```python
from build123d import *

# Parameters (mm, degrees)
F1_DEPTH = 6.3
F2_SIZE  = 0.5
F3_SIZE  = 2
F4_W     = 10
F4_H     = 0.938
F4_H_2   = 5.5
F5_DEPTH = 2.5
F6_SIZE  = 1
F7_SIZE  = 2


# Not quite as in the source:
# - a feature names something its author has since deleted; it is built from what else it names


with BuildPart() as f1:
    # F0 (on Top) → F1 (new body)
    with BuildSketch(Plane.XY):
        with BuildLine():
            ThreePointArc((27, -22.5), (49.5, 0), (27, 22.5))
            Line((27, 22.5), (27, 4))
            Line((27, 4), (34.5, 4))
            ThreePointArc((34.5, 4), (38.5, 0), (34.5, -4))
            Line((34.5, -4), (27, -4))
            Line((27, -4), (27, -22.5))
        make_face()
        with BuildLine():
            ThreePointArc((30.8505792452, -11.1005792452), (28.6005792452, -8.8505792452), (30.8505792452, -6.6005792452))
            Line((30.8505792452, -6.6005792452), (40.8505792452, -6.6005792452))
            ThreePointArc((40.8505792452, -6.6005792452), (43.1005792452, -8.8505792452), (40.8505792452, -11.1005792452))
            Line((40.8505792452, -11.1005792452), (30.8505792452, -11.1005792452))
        make_face(mode=Mode.SUBTRACT)
        with BuildLine():
            ThreePointArc((30.8505792452, 6.6005792452), (28.6005792452, 8.8505792452), (30.8505792452, 11.1005792452))
            Line((30.8505792452, 11.1005792452), (40.8505792452, 11.1005792452))
            ThreePointArc((40.8505792452, 11.1005792452), (43.1005792452, 8.8505792452), (40.8505792452, 6.6005792452))
            Line((40.8505792452, 6.6005792452), (30.8505792452, 6.6005792452))
        make_face(mode=Mode.SUBTRACT)
        with BuildLine():
            Line((27, 4), (27, 22.5))
            Line((27, 22.5), (-27, 22.5))
            Line((-27, 22.5), (-27, 8.905))
            ThreePointArc((-27, 8.905), (-20.7032141135, 6.2967858865), (-18.095, 0))
            ThreePointArc((-18.095, 0), (-20.7032141135, -6.2967858865), (-27, -8.905))
            Line((-27, -8.905), (-27, -22.5))
            Line((-27, -22.5), (27, -22.5))
            Line((27, -22.5), (27, -4))
            Line((27, -4), (19.5, -4))
            ThreePointArc((19.5, -4), (15.5, 0), (19.5, 4))
            Line((19.5, 4), (27, 4))
        make_face()
        with BuildLine():
            Line((23.1494207548, -11.1005792452), (13.1494207548, -11.1005792452))
            ThreePointArc((13.1494207548, -11.1005792452), (10.8994207548, -8.8505792452), (13.1494207548, -6.6005792452))
            Line((13.1494207548, -6.6005792452), (23.1494207548, -6.6005792452))
            ThreePointArc((23.1494207548, -6.6005792452), (25.3994207548, -8.8505792452), (23.1494207548, -11.1005792452))
        make_face(mode=Mode.SUBTRACT)
        with BuildLine():
            ThreePointArc((13.1494207548, 6.6005792452), (10.8994207548, 8.8505792452), (13.1494207548, 11.1005792452))
            Line((13.1494207548, 11.1005792452), (23.1494207548, 11.1005792452))
            ThreePointArc((23.1494207548, 11.1005792452), (25.3994207548, 8.8505792452), (23.1494207548, 6.6005792452))
            Line((23.1494207548, 6.6005792452), (13.1494207548, 6.6005792452))
        make_face(mode=Mode.SUBTRACT)
        with BuildLine():
            Line((-27, 8.905), (-27, 22.5))
            ThreePointArc((-27, 22.5), (-49.5, 0), (-27, -22.5))
            Line((-27, -22.5), (-27, -8.905))
            ThreePointArc((-27, -8.905), (-35.905, 0), (-27, 8.905))
        make_face()
    extrude(amount=F1_DEPTH)

    # F2
    f2_edges = [f1.edges().sort_by_distance(p)[0] for p in [
        (18.149421, 11.100579, 6.3),
        (35.850579, 11.100579, 6.3),
        (35.850579, -6.600579, 6.3),
        (18.149421, -6.600579, 6.3),
        (35.850579, 11.100579, 0),
        (18.149421, 11.100579, 0),
        (35.850579, -6.600579, 0),
        (18.149421, -6.600579, 0),
        (43.100579, -8.850579, 0),
        (35.850579, -11.100579, 0),
        (28.600579, -8.850579, 0),
        (43.100579, 8.850579, 0),
        (35.850579, 6.600579, 0),
        (28.600579, 8.850579, 0),
        (18.149421, 6.600579, 0),
        (10.899421, 8.850579, 0),
        (25.399421, 8.850579, 0),
        (18.149421, -11.100579, 0),
        (10.899421, -8.850579, 0),
        (25.399421, -8.850579, 0),
    ]]
    chamfer(f2_edges, length=F2_SIZE)

    # F3
    f3_edges = [f1.edges().sort_by_distance(p)[0] for p in [
        (0, -22.5, 6.3),
        (0, -22.5, 0),
    ]]
    chamfer(f3_edges, length=F3_SIZE)

    # F4 (on face) → F5 (cut)
    with BuildSketch(Plane.XY.offset(6.3)):
        with Locations((18.1494207548, 12.0695792452)):
            Rectangle(F4_W, F4_H)
        with BuildLine():
            Line((13.1494207548, 11.6005792452), (13.1494207548, 12.5385792452))
            ThreePointArc((13.1494207548, 12.5385792452), (9.4614207548, 8.8505792452), (13.1494207548, 5.1625792452))
            Line((13.1494207548, 5.1625792452), (13.1494207548, 6.1005792452))
            ThreePointArc((13.1494207548, 6.1005792452), (10.3994207548, 8.8505792452), (13.1494207548, 11.6005792452))
        make_face()
        with BuildLine():
            Line((13.1494207548, 6.1005792452), (13.1494207548, 11.6005792452))
            ThreePointArc((13.1494207548, 11.6005792452), (10.3994207548, 8.8505792452), (13.1494207548, 6.1005792452))
        make_face()
        with Locations((18.1494207548, 8.8505792452)):
            Rectangle(F4_W, F4_H_2)
        with Locations((18.1494207548, 5.6315792452)):
            Rectangle(F4_W, F4_H)
        with BuildLine():
            ThreePointArc((23.1494207548, 6.1005792452), (25.8994207548, 8.8505792452), (23.1494207548, 11.6005792452))
            Line((23.1494207548, 11.6005792452), (23.1494207548, 6.1005792452))
        make_face()
        with BuildLine():
            ThreePointArc((23.1494207548, 5.1625792452), (26.8374207548, 8.8505792452), (23.1494207548, 12.5385792452))
            Line((23.1494207548, 12.5385792452), (23.1494207548, 11.6005792452))
            ThreePointArc((23.1494207548, 11.6005792452), (25.8994207548, 8.8505792452), (23.1494207548, 6.1005792452))
            Line((23.1494207548, 6.1005792452), (23.1494207548, 5.1625792452))
        make_face()
        with BuildLine():
            ThreePointArc((30.8505792452, 12.5385792452), (27.1625792452, 8.8505792452), (30.8505792452, 5.1625792452))
            Line((30.8505792452, 5.1625792452), (30.8505792452, 6.1005792452))
            ThreePointArc((30.8505792452, 6.1005792452), (28.1005792452, 8.8505792452), (30.8505792452, 11.6005792452))
            Line((30.8505792452, 11.6005792452), (30.8505792452, 12.5385792452))
        make_face()
        with BuildLine():
            ThreePointArc((30.8505792452, 11.6005792452), (28.1005792452, 8.8505792452), (30.8505792452, 6.1005792452))
            Line((30.8505792452, 6.1005792452), (30.8505792452, 11.6005792452))
        make_face()
        with Locations((35.8505792452, 8.8505792452)):
            Rectangle(F4_W, F4_H_2)
        with Locations((35.8505792452, 12.0695792452)):
            Rectangle(F4_W, F4_H)
        with Locations((35.8505792452, 5.6315792452)):
            Rectangle(F4_W, F4_H)
        with BuildLine():
            Line((40.8505792452, 6.1005792452), (40.8505792452, 5.1625792452))
            ThreePointArc((40.8505792452, 5.1625792452), (44.5385792452, 8.8505792452), (40.8505792452, 12.5385792452))
            Line((40.8505792452, 12.5385792452), (40.8505792452, 11.6005792452))
            ThreePointArc((40.8505792452, 11.6005792452), (43.6005792452, 8.8505792452), (40.8505792452, 6.1005792452))
        make_face()
        with BuildLine():
            Line((40.8505792452, 11.6005792452), (40.8505792452, 6.1005792452))
            ThreePointArc((40.8505792452, 6.1005792452), (43.6005792452, 8.8505792452), (40.8505792452, 11.6005792452))
        make_face()
        with Locations((18.1494207548, -8.8505792452)):
            Rectangle(F4_W, F4_H_2)
        with BuildLine():
            ThreePointArc((13.1494207548, -6.1005792452), (10.3994207548, -8.8505792452), (13.1494207548, -11.6005792452))
            Line((13.1494207548, -11.6005792452), (13.1494207548, -6.1005792452))
        make_face()
        with BuildLine():
            Line((23.1494207548, -6.1005792452), (23.1494207548, -11.6005792452))
            ThreePointArc((23.1494207548, -11.6005792452), (25.8994207548, -8.8505792452), (23.1494207548, -6.1005792452))
        make_face()
        with Locations((18.1494207548, -5.6315792452)):
            Rectangle(F4_W, F4_H)
        with BuildLine():
            Line((23.1494207548, -11.6005792452), (23.1494207548, -12.5385792452))
            ThreePointArc((23.1494207548, -12.5385792452), (26.8374207548, -8.8505792452), (23.1494207548, -5.1625792452))
            Line((23.1494207548, -5.1625792452), (23.1494207548, -6.1005792452))
            ThreePointArc((23.1494207548, -6.1005792452), (25.8994207548, -8.8505792452), (23.1494207548, -11.6005792452))
        make_face()
        with Locations((18.1494207548, -12.0695792452)):
            Rectangle(F4_W, F4_H)
        with BuildLine():
            ThreePointArc((13.1494207548, -5.1625792452), (9.4614207548, -8.8505792452), (13.1494207548, -12.5385792452))
            Line((13.1494207548, -12.5385792452), (13.1494207548, -11.6005792452))
            ThreePointArc((13.1494207548, -11.6005792452), (10.3994207548, -8.8505792452), (13.1494207548, -6.1005792452))
            Line((13.1494207548, -6.1005792452), (13.1494207548, -5.1625792452))
        make_face()
        with BuildLine():
            ThreePointArc((30.8505792452, -5.1625792452), (27.1625792452, -8.8505792452), (30.8505792452, -12.5385792452))
            Line((30.8505792452, -12.5385792452), (30.8505792452, -11.6005792452))
            ThreePointArc((30.8505792452, -11.6005792452), (28.1005792452, -8.8505792452), (30.8505792452, -6.1005792452))
            Line((30.8505792452, -6.1005792452), (30.8505792452, -5.1625792452))
        make_face()
        with Locations((35.8505792452, -5.6315792452)):
            Rectangle(F4_W, F4_H)
        with Locations((35.8505792452, -8.8505792452)):
            Rectangle(F4_W, F4_H_2)
        with Locations((35.8505792452, -12.0695792452)):
            Rectangle(F4_W, F4_H)
        with BuildLine():
            ThreePointArc((30.8505792452, -6.1005792452), (28.1005792452, -8.8505792452), (30.8505792452, -11.6005792452))
            Line((30.8505792452, -11.6005792452), (30.8505792452, -6.1005792452))
        make_face()
        with BuildLine():
            Line((40.8505792452, -6.1005792452), (40.8505792452, -11.6005792452))
            ThreePointArc((40.8505792452, -11.6005792452), (43.6005792452, -8.8505792452), (40.8505792452, -6.1005792452))
        make_face()
        with BuildLine():
            Line((40.8505792452, -11.6005792452), (40.8505792452, -12.5385792452))
            ThreePointArc((40.8505792452, -12.5385792452), (44.5385792452, -8.8505792452), (40.8505792452, -5.1625792452))
            Line((40.8505792452, -5.1625792452), (40.8505792452, -6.1005792452))
            ThreePointArc((40.8505792452, -6.1005792452), (43.6005792452, -8.8505792452), (40.8505792452, -11.6005792452))
        make_face()
    extrude(amount=-F5_DEPTH, mode=Mode.SUBTRACT)

    # F6
    f6_edges = [f1.edges().sort_by_distance(p)[0] for p in [
        (10.899421, 8.850579, 3.8),
        (18.149421, 6.600579, 3.8),
        (25.399421, 8.850579, 3.8),
        (18.149421, 11.100579, 3.8),
        (35.850579, 11.100579, 3.8),
        (28.600579, 8.850579, 3.8),
        (43.100579, 8.850579, 3.8),
        (35.850579, 6.600579, 3.8),
        (35.850579, -6.600579, 3.8),
        (28.600579, -8.850579, 3.8),
        (43.100579, -8.850579, 3.8),
        (35.850579, -11.100579, 3.8),
        (18.149421, -6.600579, 3.8),
        (10.899421, -8.850579, 3.8),
        (25.399421, -8.850579, 3.8),
        (18.149421, -11.100579, 3.8),
    ]]
    chamfer(f6_edges, length=F6_SIZE)

    # F7
    f7_edges = [f1.edges().sort_by_distance(p)[0] for p in [
        (27, 4, 0),
        (38.5, 0, 0),
        (27, -4, 0),
        (15.5, 0, 0),
    ]]
    chamfer(f7_edges, length=F7_SIZE)


solid = f1.part
```
Model file for the job. Use its own axes, mm. A direction names the side the tool comes from. Give positions to 0.01 mm unless a question says otherwise; leave off trailing zeros. Order: outer loops, then holes, each group sorted by start corner. A loop starts at its lowest first (then second) coordinate and runs counter-clockwise, first axis right, second up.
1) Saw through at A-A, the plane z = 5.25. Write the cut outline in (x, y) (3 decimals).
2) Wall check: probe 1 along X at (y, z) = (-10.5, 4.5); probe 2 along Y at (x, z) = (33, 6.25); probe 3 along X at (y, z) = (-11, 6.25). Give the ranges that are in metal, low to high.
3) Pin check, flat tips, straight feed: pin 1 (0.8 mm diameter, centred on x = 20, z = 5, fed in from +Y); pin 2 (6 mm diameter, centred on x = 17, y = 9, fed in from +Z); pin 3 (3.5 mm diameter, centred on x = 36, y = -10, fed in from +Z). Stop position of each tip, or through.
4) Mould opens along X. For faces 5 (the flat face through (18, 11.101, 2)), 6 (the cylindrical face through (38.5, 0.1, 4.1)), 7 (the flat face through (-1, 0, 6.3)), 8 (the conical face through (47.62, -0.454, 0.125)) say: +X half, -X half, draft (parallel to the pull), parting line (faces both ways), or undercut.
5) Saw through at B-B, the plane x = -25. Write the cut outline in (y, z).
6) 3-axis set-ups, long thin cutter, end or side, ignore diameter. For faces 1 (the flat face through (18, -5.163, 5)), 2 (the flat face through (0, -22.5, 3)), 3 (the conical face through (38.8, 0.1, 1.7)), 4 (the cylindrical face through (43.1, 8.9, 1.6)): which of +Z, -Z, +X, -X, +Y, -Y reach the whole face in a straight line?
7) Saw through at C-C, the plane x = 35.5. Count the separate pieces of the cut face and the enclosed holes in it, then the cut area to 3 significant figures.
Computed:
1. outline: (-27, -21.55) - (27, -21.55) arc R21.55 ccw to (27, 21.55) - (-27, 21.55) arc R21.55 ccw to start; hole circle Ø17.81 at (-27, 0); hole (13.149, -12.539) - (23.149, -12.539) arc R3.688 ccw to (23.149, -5.163) - (13.149, -5.163) arc R3.688 ccw to start; hole (13.149, 5.163) - (23.149, 5.163) arc R3.688 ccw to (23.149, 12.539) - (13.149, 12.539) arc R3.688 ccw to start; hole (19.5, -4) - (34.5, -4) arc R4 ccw to (34.5, 4) - (19.5, 4) arc R4 ccw to start; hole (30.851, -12.539) - (40.851, -12.539) arc R3.688 ccw to (40.851, -5.163) - (30.851, -5.163) arc R3.688 ccw to start; hole (30.851, 5.163) - (40.851, 5.163) arc R3.688 ccw to (40.851, 12.539) - (30.851, 12.539) arc R3.688 ccw to start
2. probe 1: x = -46.67 to 9.85, 26.45 to 27.55, 44.15 to 46.67
2. probe 2: y = -19.65 to -12.54, -5.16 to -4, 4 to 5.16, 12.54 to 19.65
2. probe 3: x = -44.36 to 10.15, 26.15 to 27.85, 43.85 to 44.36
3. pin 1: stops at y = 22.2
3. pin 2: stops at z = 3.7
3. pin 3: stops at z = 3.45
4. face 5: undercut
4. face 6: undercut
4. face 7: draft
4. face 8: +X half
5. outline: (-22.5, 2) - (-20.5, 0) - (-8.68, 0) - (-8.68, 6.3) - (-20.5, 6.3) - (-22.5, 4.3) - close; (8.68, 0) - (20.5, 0) - (22.5, 2) - (22.5, 4.3) - (20.5, 6.3) - (8.68, 6.3) - close
6. face 1: +Z
6. face 2: +Z, -Z, +X, -X, -Y
6. face 3: -Z
6. face 4: +Z, -Z
7. separate pieces: 4
7. enclosed holes: 0
7. area: 127 mm2
